For this review, take the finished solid that the model builds, in its own axes (mm). A direction names the side the tool comes from. Round coordinates to 2 decimals unless told otherwise and drop trailing zeros. Order: outer loops, then holes, each group sorted by start corner. A loop starts at its lowest first (then second) coordinate and runs counter-clockwise, first axis right, second up. Notation, with made-up numbers: (22, -19.75) - (32, -19.75) arc R30 cw to (32, 7.25) - close; hole circle Ø6 at (-23.5, -4). An arc over 180 degrees is marked (long way). One line per question, with ' | ' between items.
```python
from build123d import *

# Parameters (mm, degrees)
SKETCH4_W          = 2.5
SKETCH4_H          = 2.5
CUT_EXTRUDE1_DEPTH = 20


with BuildPart() as part:
    # Sketch2 → Revolve1 (revolve)
    with BuildSketch(Plane.XY, mode=Mode.PRIVATE) as revolve1_sk:
        Polygon((11, 0), (17.5, 0), (17.5, -3), (19.5, -3), (19.5, 0), (22.5, 0), (22.5, 6), (16, 6), (16, 32), (11, 32), (11, 6), align=None)
    revolve(revolve1_sk.sketch.rotate(Axis((0, 28.805193162, 0), (0, 1, 0)), 270), axis=Axis((0, 28.805193162, 0), (0, 1, 0)))

    # Sketch4 → Cut-Extrude1 (cut)
    with BuildSketch(Plane.XY):
        with Locations((0, 13.522413215)):
            Rectangle(SKETCH4_W, SKETCH4_H)
        with Locations((0, 7.522413215)):
            Rectangle(SKETCH4_W, SKETCH4_H)
        with Locations((0, 19.522413215)):
            Rectangle(SKETCH4_W, SKETCH4_H)
        with Locations((0, 25.522413215)):
            Rectangle(SKETCH4_W, SKETCH4_H)
    extrude(amount=-CUT_EXTRUDE1_DEPTH, mode=Mode.SUBTRACT)


solid = part.part
```
(1) Mouldability with a two-part tool opening along Y and no side actions: class faces 4 (the flat face through (0, 26.772, -13)), 5 (the cylindrical face through (19.334, -1.479, -2.539)), 6 (the flat face through (10, 0, 17)) as released by +Y, released by -Y, zero draft, split by the parting line, or undercut.
Output values:
face 4: undercut | face 5: zero draft | face 6: released by -Y
(2) We need section D-D on y = 28. State the section outline as (x, z) points.
Output values:
outline: circle Ø32 at (0, 0); hole circle Ø22 at (0, 0)
(3) We need section B-B on x = -7. State the section outline as (y, z) points, plus the area to 3 significant figures.
Output values:
outline: (-3, -18.2) - (0, -18.2) - (0, -21.38) - (6, -21.38) - (6, -14.39) - (32, -14.39) - (32, -8.49) - (0, -8.49) - (0, -16.04) - (-3, -16.04) - close; (-3, 16.04) - (0, 16.04) - (0, 8.49) - (32, 8.49) - (32, 14.39) - (6, 14.39) - (6, 21.38) - (0, 21.38) - (0, 18.2) - (-3, 18.2) - close | area: 475 mm^2
(4) We need section C-C on x = 0. Give the number of separate pieces and of enclosed holes in the cut face, plus the area to 3 significant figures.
Output values:
separate pieces: 6 | enclosed holes: 0 | area: 360 mm^2
(5) Insertion check: pin 1 (4 mm diameter, centred on x = -0.5, y = 16.5, fed in from +Z); pin 2 (3 mm diameter, centred on y = 7, z = -14.5, fed in from -X); pin 3 (1.5 mm diameter, centred on x = 10.5, y = 19.5, fed in from -Z). Each pin has a flat end and moves straight along its axis. Give the tip position at first contact, or say it passes through.
Output values:
pin 1: z = 16 | pin 2: x = -18.09 | pin 3: z = -12.69
(6) For faces 1 (the cylindrical face through (-6.13, 19.18, 14.78)), 2 (the flat face through (1.25, 26, -13)), 3 (the cylindrical face through (-8.618, 3.042, 20.784)), list the 3-axis set-ups (+Z, -Z, +X, -X, +Y, -Y) from which the entire face can be reached by the end or side of a thin tool; tool diameter is ignored.
Output values:
face 1: +Y | face 2: -Z | face 3: +Y, -Y
(7) For probe 1 along X at (y, z) = (11, -0.5); probe 2 along X at (y, z) = (-2, 0); probe 3 along Y at (x, z) = (1.5, -15.5), list the stretches that pass through material, from the lowest coordinate up. Write a range as [from, to].
Output values:
probe 1: [-15.99, -10.99], [10.99, 15.99] | probe 2: [-19.5, -17.5], [17.5, 19.5] | probe 3: [0, 32]
(8) We need section A-A on z = 0. State the section outline as (x, y) points.
Output values:
outline: (-22.5, 0) - (-19.5, 0) - (-19.5, -3) - (-17.5, -3) - (-17.5, 0) - (-11, 0) - (-11, 32) - (-16, 32) - (-16, 6) - (-22.5, 6) - close; (11, 0) - (17.5, 0) - (17.5, -3) - (19.5, -3) - (19.5, 0) - (22.5, 0) - (22.5, 6) - (16, 6) - (16, 32) - (11, 32) - close
